Input: part model. Units: mm. Frame: model coordinates. Give positions to 0.01 mm unless a question says otherwise; leave off trailing zeros. Write each loop counter-clockwise with the first axis right and the second up, starting at its lowest first coordinate (ties: lowest second). Pieces come first, ordered by that corner, then holes. Notation, with made-up numbers: (24, 67) -> (78, 67) arc R9 ccw to (78, 74) -> close; hole circle Ø2 at (37, -14.75). An arc over 180 degrees is marked (long way). Return JSON: item names as keys, results as strings. Group by question number.
Item 1: Mould query, pull axis X, two halves, no side actions, for faces 1 (the face through (21.5, 8.3, 1.3)), 2 (the face through (101.6, 24, 1)), 3 (the face through (67, 6.35, 1)). Classes: released by +X, released by -X, zero draft, split by the parting line, or undercut.
Item 2: Section A-A, the plane x = 37. Return loops of the section in (y, z), then the cut area to 3 significant figures.
Item 3: Section B-B, the plane y = 23.5. Return loops of the section in (x, z), then the cut area to 3 significant figures.
Item 4: Section D-D, the plane x = 74. Return loops of the section in (y, z), then the cut area to 3 significant figures.
Item 5: Line query: line 1 (X direction, y = 44, z = 1.25); line 2 (X direction, y = 27.5, z = 0.4); line 3 (Y direction, x = 57, z = 0.7). Output: solid intervals per line, ascending. Write a range as [from, to].
Item 6: Section C-C, the plane y = 32. Return loops of the section in (x, z) (3 decimals).
Item 7: Pin query (flat end, axial travel): P1, Ø3, axis at x = 95.25, y = 43.18, coming from the +Z side. Return the tip coordinate at first contact, or that it passes through.
from build123d import *

# Parameters (mm, degrees)
SKETCH1_R           = 1.75006
SKETCH1_R_2         = 1.750059992
BOSS_EXTRUDE1_DEPTH = 2.54


with BuildPart() as part:
    # Sketch1 → Boss-Extrude1 (new body)
    with BuildSketch(Plane.XY):
        Polygon((2.54, 0), (99.06, 0), (101.6, 0), (101.6, 2.54), (101.6, 46.99), (101.6, 49.53), (99.06, 49.53), (2.54, 49.53), (0, 49.53), (0, 46.99), (0, 2.54), (0, 0), align=None)
        with Locations((6.35, 43.18)):
            Circle(SKETCH1_R, mode=Mode.SUBTRACT)
        with Locations(Location((6.35, 6.35, 0), (0, 0, 180))):
            Circle(SKETCH1_R, mode=Mode.SUBTRACT)
        with Locations((95.25, 6.35)):
            Circle(SKETCH1_R, mode=Mode.SUBTRACT)
        with Locations(Location((95.25, 43.18, 0), (0, 0, 180))):
            Circle(SKETCH1_R_2, mode=Mode.SUBTRACT)
        with BuildLine():
            Line((22.882222071, 38.345496006), (43.995572894, 28.320908231))
            ThreePointArc((43.995572894, 28.320908231), (46.442286843, 28.46846732), (47.625, 30.615412225))
            Line((47.625, 30.615412225), (47.625, 40.64))
            ThreePointArc((47.625, 40.64), (46.881051224, 42.436051224), (45.085, 43.18))
            Line((45.085, 43.18), (23.971649177, 43.18))
            ThreePointArc((23.971649177, 43.18), (21.493783145, 41.19837257), (22.882222071, 38.345496006))
        make_face(mode=Mode.SUBTRACT)
        with BuildLine():
            Line((47.625, 18.914587775), (47.625, 8.89))
            ThreePointArc((47.625, 8.89), (46.881051224, 7.093948776), (45.085, 6.35))
            Line((45.085, 6.35), (23.971649177, 6.35))
            ThreePointArc((23.971649177, 6.35), (21.493783145, 8.33162743), (22.882222071, 11.184503994))
            Line((22.882222071, 11.184503994), (43.995572894, 21.209091769))
            ThreePointArc((43.995572894, 21.209091769), (46.442286843, 21.06153268), (47.625, 18.914587775))
        make_face(mode=Mode.SUBTRACT)
        with BuildLine():
            Line((78.717777929, 11.184503994), (57.604427106, 21.209091769))
            ThreePointArc((57.604427106, 21.209091769), (55.157713157, 21.06153268), (53.975, 18.914587775))
            Line((53.975, 18.914587775), (53.975, 8.89))
            ThreePointArc((53.975, 8.89), (54.718948776, 7.093948776), (56.515, 6.35))
            Line((56.515, 6.35), (77.628350823, 6.35))
            ThreePointArc((77.628350823, 6.35), (80.106216855, 8.33162743), (78.717777929, 11.184503994))
        make_face(mode=Mode.SUBTRACT)
        with BuildLine():
            Line((53.975, 30.615412225), (53.975, 40.64))
            ThreePointArc((53.975, 40.64), (54.718948776, 42.436051224), (56.515, 43.18))
            Line((56.515, 43.18), (77.628350823, 43.18))
            ThreePointArc((77.628350823, 43.18), (80.106216855, 41.19837257), (78.717777929, 38.345496006))
            Line((78.717777929, 38.345496006), (57.604427106, 28.320908231))
            ThreePointArc((57.604427106, 28.320908231), (55.157713157, 28.46846732), (53.975, 30.615412225))
        make_face(mode=Mode.SUBTRACT)
        with BuildLine():
            Line((9.979427106, 37.442318053), (31.847258551, 27.059503994))
            ThreePointArc((31.847258551, 27.059503994), (33.297831444, 24.765), (31.847258551, 22.470496006))
            Line((31.847258551, 22.470496006), (9.979427106, 12.087681947))
            ThreePointArc((9.979427106, 12.087681947), (7.532713157, 12.235241036), (6.35, 14.382185941))
            Line((6.35, 14.382185941), (6.35, 35.147814059))
            ThreePointArc((6.35, 35.147814059), (7.532713157, 37.294758964), (9.979427106, 37.442318053))
        make_face(mode=Mode.SUBTRACT)
        with BuildLine():
            Line((91.620572894, 12.087681947), (69.752741449, 22.470496006))
            ThreePointArc((69.752741449, 22.470496006), (68.302168556, 24.765), (69.752741449, 27.059503994))
            Line((69.752741449, 27.059503994), (91.620572894, 37.442318053))
            ThreePointArc((91.620572894, 37.442318053), (94.067286843, 37.294758964), (95.25, 35.147814059))
            Line((95.25, 35.147814059), (95.25, 14.382185941))
            ThreePointArc((95.25, 14.382185941), (94.067286843, 12.235241036), (91.620572894, 12.087681947))
        make_face(mode=Mode.SUBTRACT)
    extrude(amount=BOSS_EXTRUDE1_DEPTH)


solid = part.part
Answer below:
{
 "1": {"face 1": "undercut", "face 2": "released by +X", "face 3": "undercut"},
 "2": {"outline": "(0, 0) -> (6.35, 0) -> (6.35, 2.54) -> (0, 2.54) -> close; (17.89, 0) -> (31.64, 0) -> (31.64, 2.54) -> (17.89, 2.54) -> close; (43.18, 0) -> (49.53, 0) -> (49.53, 2.54) -> (43.18, 2.54) -> close", "area": "67.2 mm2"},
 "3": {"outline": "(0, 0) -> (6.35, 0) -> (6.35, 2.54) -> (0, 2.54) -> close; (32.96, 0) -> (68.64, 0) -> (68.64, 2.54) -> (32.96, 2.54) -> close; (95.25, 0) -> (101.6, 0) -> (101.6, 2.54) -> (95.25, 2.54) -> close", "area": "123 mm2"},
 "4": {"outline": "(0, 0) -> (6.35, 0) -> (6.35, 2.54) -> (0, 2.54) -> close; (13.42, 0) -> (20.45, 0) -> (20.45, 2.54) -> (13.42, 2.54) -> close; (29.08, 0) -> (36.11, 0) -> (36.11, 2.54) -> (29.08, 2.54) -> close; (43.18, 0) -> (49.53, 0) -> (49.53, 2.54) -> (43.18, 2.54) -> close", "area": "68.0 mm2"},
 "5": {"line 1": "x = [0, 4.8], [7.9, 93.7], [96.8, 101.6]", "line 2": "x = [0, 6.35], [30.92, 70.68], [95.25, 101.6]", "line 3": "y = [0, 6.35], [21.41, 28.12], [43.18, 49.53]"},
 "6": {"outline": "(0, 0) -> (6.35, 0) -> (6.35, 2.54) -> (0, 2.54) -> close; (21.442, 0) -> (36.247, 0) -> (36.247, 2.54) -> (21.442, 2.54) -> close; (47.625, 0) -> (53.975, 0) -> (53.975, 2.54) -> (47.625, 2.54) -> close; (65.353, 0) -> (80.158, 0) -> (80.158, 2.54) -> (65.353, 2.54) -> close; (95.25, 0) -> (101.6, 0) -> (101.6, 2.54) -> (95.25, 2.54) -> close"},
 "7": {"P1": "passes through"}
}
